```python
from build123d import *

# Parameters (mm, degrees)
EXTRUDE_1_DEPTH = 15.5
SHELL_1_T       = -2
FILLET_1_R      = 1


with BuildPart() as part:
    # Эскиз2 → Бобышка-Вытянуть1 (new body)
    with BuildSketch(Plane(origin=(0, 0, 0), x_dir=(1, 0, 0), z_dir=(0, 1, 0))):
        with BuildLine():
            Line((-7, 0), (-76, 0))
            ThreePointArc((-76, 0), (-80.949747468, 2.050252532), (-83, 7))
            Line((-83, 7), (-83, 175))
            ThreePointArc((-83, 175), (-80.949747468, 179.949747468), (-76, 182))
            Line((-76, 182), (-7, 182))
            ThreePointArc((-7, 182), (-2.050252532, 179.949747468), (0, 175))
            Line((0, 175), (0, 7))
            ThreePointArc((0, 7), (-2.050252532, 2.050252532), (-7, 0))
        make_face()
    extrude(amount=EXTRUDE_1_DEPTH)

    # Оболочка1
    shell_1_openings = [part.faces().sort_by_distance(p)[0] for p in [
        (-41.5, 0, -91),
    ]]
    offset(amount=SHELL_1_T, openings=shell_1_openings, kind=Kind.INTERSECTION)

    # Скругление1
    fillet_1_edges = [part.edges().sort_by_distance(p)[0] for p in [
        (-2.050252532, 15.5, -179.949747468),
        (-41.5, 15.5, -182),
        (-80.949747468, 15.5, -179.949747468),
        (-83, 15.5, -91),
        (-80.949747468, 15.5, -2.050252532),
        (-41.5, 15.5, 0),
        (-2.050252532, 15.5, -2.050252532),
        (0, 15.5, -91),
    ]]
    fillet(fillet_1_edges, radius=FILLET_1_R)


solid = part.part
```
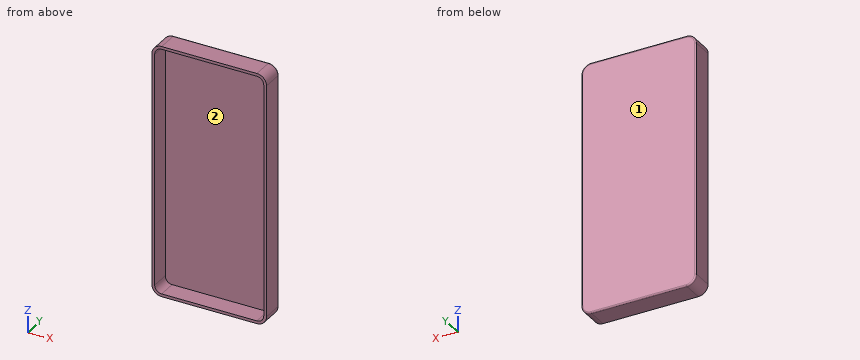
CAD build for the part. Positions are in the model's coordinates, mm. Face numbers are marked on the shaded views. Coordinates: 2 decimals unless noted, no trailing zeros. Write each loop counter-clockwise with the first axis right and the second up, starting at its lowest first coordinate (ties: lowest second). Pieces come first, ordered by that corner, then holes. Notation, with made-up numbers: (-27, 29.25) -> (-18, 29.25) arc R28 cw to (-18, 67.25) -> close; hole circle Ø3 at (3, 53). An arc over 180 degrees is marked (long way). Return JSON: item names as keys, results as strings. Group by question number.
Q1. Pull direction X, two halves, no side cores. Call the marked faces 1 and 2: released by +X, released by -X, zero draft, split by the parting line, or undercut.
Q2. Cut at A-A, the plane y = 9.5. Give the cut face in (x, z).
Q3. Drill centre lines: line 1 (Z direction, x = -33, y = 7); line 2 (X direction, y = 3.25, z = -164.5); line 3 (Y direction, x = -76.5, z = -161). Where is each one in solid material? Low to high.
Q4. Cut at B-B, the plane z = -54.5. Give the cut face in (x, y), then the cut area to 3 significant figures.
Q5. Cut at C-C, the plane x = -69.5. Give the cut face in (y, z), then the cut area to 3 significant figures.
Q6. Flat gauge pin, fed straight in: pin 1 (1.5 mm diameter, centred on x = -57, z = -47, fed in from -Y). Where does the tip first touch, or does it go through?
Returned:
{
 "1": {"face 1": "zero draft", "face 2": "undercut"},
 "2": {"outline": "(-83, -175) arc R7 ccw to (-76, -182) -> (-7, -182) arc R7 ccw to (0, -175) -> (0, -7) arc R7 ccw to (-7, 0) -> (-76, 0) arc R7 ccw to (-83, -7) -> close; hole (-81, -175) arc R5 ccw to (-76, -180) -> (-7, -180) arc R5 ccw to (-2, -175) -> (-2, -7) arc R5 ccw to (-7, -2) -> (-76, -2) arc R5 ccw to (-81, -7) -> close"},
 "3": {"line 1": "z = -182 to -180, -2 to 0", "line 2": "x = -83 to -81, -2 to 0", "line 3": "y = 13.5 to 15.5"},
 "4": {"outline": "(-83, 0) -> (-81, 0) -> (-81, 13.5) -> (-2, 13.5) -> (-2, 0) -> (0, 0) -> (0, 14.5) arc R1 ccw to (-1, 15.5) -> (-82, 15.5) arc R1 ccw to (-83, 14.5) -> close", "area": "220 mm2"},
 "5": {"outline": "(0, -182) -> (14.5, -182) arc R1 ccw to (15.5, -181) -> (15.5, -1) arc R1 ccw to (14.5, 0) -> (0, 0) -> (0, -2) -> (13.5, -2) -> (13.5, -180) -> (0, -180) -> close", "area": "418 mm2"},
 "6": {"pin 1": "stops at y = 13.5"}
}
